```python
from build123d import *

# Parameters (mm, degrees)
SKETCH_1_W                  = 57.4
SKETCH_1_H                  = 28.5
EXTRUDE_1_DEPTH             = 12
SKETCH_2_W                  = 57.4
SKETCH_2_H                  = 26
EXTRUDE_2_DEPTH             = 19
SKETCH_3_W                  = 16.1
SKETCH_3_H                  = 20.5
CUT_EXTRUDE_1_DEPTH         = 7.7
SKETCH_4_W                  = 28.1
SKETCH_4_H                  = 20.5
CUT_EXTRUDE_2_DEPTH         = 41.7
SKETCH_5_W                  = 31
SKETCH_5_H                  = 20.5
CUT_EXTRUDE_3_DEPTH         = 0.3
CUT_EXTRUDE_4_DEPTH         = 2.9
SKETCH_7_W                  = 12
SKETCH_7_H                  = 2.5
CUT_EXTRUDE_5_DEPTH         = 46.4
CUT_EXTRUDE_6_DEPTH         = 7.7
CUT_EXTRUDE_7_DEPTH         = 14.1
CUT_EXTRUDE_8_DEPTH         = 3.3
SKETCH_11_W                 = 11
SKETCH_11_H                 = 12
EXTRUDE_3_DEPTH             = 2.5
SKETCH_12_W                 = 12
SKETCH_12_H                 = 2.75
EXTRUDE_4_DEPTH             = 6
SKETCH_13_W                 = 6
SKETCH_13_H                 = 12
EXTRUDE_5_DEPTH             = 2.5
SKETCH_14_W                 = 12
SKETCH_14_H                 = 5.25
EXTRUDE_6_DEPTH             = 6
SKETCH_15_W                 = 5
SKETCH_15_H                 = 2.5
CUT_EXTRUDE_9_DEPTH         = 45.999333328
SKETCH_16_W                 = 5
SKETCH_16_H                 = 2.5
CUT_EXTRUDE_10_DEPTH        = 45.999333328
SKETCH_17_W                 = 5
SKETCH_17_H                 = 26
EXTRUDE_7_DEPTH             = 2
SKETCH_18_W                 = 10
SKETCH_18_H                 = 6
EXTRUDE_8_DEPTH             = 7
SKETCH_19_W                 = 4
SKETCH_19_H                 = 6.5
HOLE_WIZARD_3_5_3_5_1_D     = 3.5
HOLE_WIZARD_3_5_3_5_1_DEPTH = 12
HOLE_WIZARD_3_5_3_5_2_D     = 3.5
HOLE_WIZARD_3_0_3_3_D       = 3
HOLE_WIZARD_3_0_3_3_DEPTH   = 37.5
HOLE_WIZARD_3_5_3_5_3_D     = 3.5
FILLET_1_R                  = 7
EXTRUDE_START               = -19
SKETCH_28_W                 = 6
SKETCH_28_H                 = 5.25
SKETCH_28_R                 = 1.75
EXTRUDE_9_DEPTH             = 7


with BuildPart() as part:
    # Эскиз1 → Бобышка-Вытянуть1 (new body)
    with BuildSketch(Plane.XY.offset(12)):
        with Locations((0, 1.25)):
            Rectangle(SKETCH_1_W, SKETCH_1_H)
    extrude(amount=-EXTRUDE_1_DEPTH)

    # Эскиз2 → Бобышка-Вытянуть2 (add)
    with BuildSketch(Plane.XY.offset(12)):
        Rectangle(SKETCH_2_W, SKETCH_2_H)
    extrude(amount=EXTRUDE_2_DEPTH)

    # Эскиз3 → Вырез-Вытянуть1 (cut)
    with BuildSketch(Plane.ZY.offset(28.7)):
        with Locations((20.05, 0)):
            Rectangle(SKETCH_3_W, SKETCH_3_H)
    extrude(amount=-CUT_EXTRUDE_1_DEPTH, mode=Mode.SUBTRACT)

    # Эскиз4 → Вырез-Вытянуть2 (cut)
    with BuildSketch(Plane.ZY.offset(21)):
        with Locations((14.05, 0)):
            Rectangle(SKETCH_4_W, SKETCH_4_H)
    extrude(amount=-CUT_EXTRUDE_2_DEPTH, mode=Mode.SUBTRACT)

    # Эскиз5 → Вырез-Вытянуть3 (cut)
    with BuildSketch(Plane.ZY.offset(-20.7)):
        with Locations((15.5, 0)):
            Rectangle(SKETCH_5_W, SKETCH_5_H)
    extrude(amount=-CUT_EXTRUDE_3_DEPTH, mode=Mode.SUBTRACT)

    # Эскиз6 → Вырез-Вытянуть4 (cut)
    with BuildSketch(Plane.XY.offset(31)):
        Polygon((28.7, -13), (28.7, 13), (20.7, 13), (20.7, 10.25), (21, 10.25), (21, -10.25), (20.7, -10.25), (20.7, -13), align=None)
    extrude(amount=-CUT_EXTRUDE_4_DEPTH, mode=Mode.SUBTRACT)

    # Эскиз7 → Вырез-Вытянуть5 (cut)
    with BuildSketch(Plane(origin=(28.7, 0, 0), x_dir=(0, 0, -1), z_dir=(1, 0, 0))):
        with Locations((-6, 14.25)):
            Rectangle(SKETCH_7_W, SKETCH_7_H)
    extrude(amount=-CUT_EXTRUDE_5_DEPTH, mode=Mode.SUBTRACT)

    # Эскиз8 → Вырез-Вытянуть6 (cut)
    with BuildSketch(Plane.ZY.offset(28.7)):
        Polygon((12, -13), (31, -13), (31, 13), (12, 13), (12, 10.25), (28.1, 10.25), (28.1, -10.25), (12, -10.25), align=None)
    extrude(amount=-CUT_EXTRUDE_6_DEPTH, mode=Mode.SUBTRACT)

    # Эскиз9 → Вырез-Вытянуть7 (cut)
    with BuildSketch(Plane.XY.offset(28.1)):
        Polygon((28.7, -13), (28.7, 13), (20.7, 13), (20.7, 10.25), (21, 10.25), (21, -10.25), (20.7, -10.25), (20.7, -13), align=None)
    extrude(amount=-CUT_EXTRUDE_7_DEPTH, mode=Mode.SUBTRACT)

    # Эскиз10 → Вырез-Вытянуть8 (cut)
    with BuildSketch(Plane.ZY.offset(21)):
        Polygon((12, -13), (31, -13), (31, 13), (12, 13), (12, 10.25), (28.1, 10.25), (28.1, -10.25), (12, -10.25), align=None)
    extrude(amount=-CUT_EXTRUDE_8_DEPTH, mode=Mode.SUBTRACT)

    # Эскиз11 → Бобышка-Вытянуть3 (add)
    with BuildSketch(Plane.XZ.offset(13)):
        with Locations((-23.2, 6)):
            Rectangle(SKETCH_11_W, SKETCH_11_H)
    extrude(amount=EXTRUDE_3_DEPTH)

    # Эскиз12 → Бобышка-Вытянуть4 (add)
    with BuildSketch(Plane.ZY.offset(17.7)):
        with Locations((25, -11.625)):
            Rectangle(SKETCH_12_W, SKETCH_12_H)
    extrude(amount=EXTRUDE_4_DEPTH)

    # Эскиз13 → Бобышка-Вытянуть5 (add)
    with BuildSketch(Plane.XZ.offset(13)):
        with Locations((-20.7, 25)):
            Rectangle(SKETCH_13_W, SKETCH_13_H)
    extrude(amount=EXTRUDE_5_DEPTH)

    # Эскиз14 → Бобышка-Вытянуть6 (add)
    with BuildSketch(Plane.ZY.offset(17.7)):
        with Locations((25, 12.875)):
            Rectangle(SKETCH_14_W, SKETCH_14_H)
    extrude(amount=EXTRUDE_6_DEPTH)

    # Эскиз15 → Вырез-Вытянуть9 (cut, through all)
    with BuildSketch(Plane(origin=(0, 0, 0), x_dir=(-1, 0, 0), z_dir=(0, 0, -1))):
        with Locations((26.2, -14.25)):
            Rectangle(SKETCH_15_W, SKETCH_15_H)
    extrude(amount=-CUT_EXTRUDE_9_DEPTH, mode=Mode.SUBTRACT)

    # Эскиз16 → Вырез-Вытянуть10 (cut, through all)
    with BuildSketch(Plane(origin=(0, 0, 0), x_dir=(-1, 0, 0), z_dir=(0, 0, -1))):
        with Locations((26.2, 14.25)):
            Rectangle(SKETCH_16_W, SKETCH_16_H)
    extrude(amount=-CUT_EXTRUDE_10_DEPTH, mode=Mode.SUBTRACT)

    # Эскиз17 → Бобышка-Вытянуть7 (add)
    with BuildSketch(Plane.XY.offset(12)):
        with Locations((-26.2, 0)):
            Rectangle(SKETCH_17_W, SKETCH_17_H)
    extrude(amount=EXTRUDE_7_DEPTH)

    # Эскиз18 → Бобышка-Вытянуть8 (add)
    with BuildSketch(Plane.ZY.offset(28.7)):
        with Locations((5, 0)):
            Rectangle(SKETCH_18_W, SKETCH_18_H)
    extrude(amount=EXTRUDE_8_DEPTH)

    # Эскиз19 → Повернуть1 (revolve)
    with BuildSketch(Plane.XZ, mode=Mode.PRIVATE) as revolve_1_sk:
        with Locations((12.2, 34.25)):
            Rectangle(SKETCH_19_W, SKETCH_19_H)
    revolve(revolve_1_sk.sketch.rotate(Axis((10.2, 0, 37.5), (0, 0, -1)), 180), axis=Axis((10.2, 0, 37.5), (0, 0, -1)))

    # Диаметр отверстия Ø3.5 (3.5)1
    with Locations(Plane.XY.offset(31)):
        with Locations((-20.7, 13), (-20.7, -13)):
            Hole(HOLE_WIZARD_3_5_3_5_1_D / 2, depth=HOLE_WIZARD_3_5_3_5_1_DEPTH)

    # Диаметр отверстия Ø3.5 (3.5)2 (through all)
    with Locations(Plane(origin=(0, 0, 0), x_dir=(-1, 0, 0), z_dir=(0, 0, -1))):
        with Locations((32.7, 0)):
            Hole(HOLE_WIZARD_3_5_3_5_2_D / 2)

    # Диаметр отверстия Ø3.0 (3)3
    with Locations(Plane(origin=(0, 0, 0), x_dir=(-1, 0, 0), z_dir=(0, 0, -1))):
        with Locations((-25.5, -5), (-25.5, 5), (25.5, -5), (25.5, 5)):
            Hole(HOLE_WIZARD_3_0_3_3_D / 2, depth=HOLE_WIZARD_3_0_3_3_DEPTH)

    # Диаметр отверстия Ø3.5 (3.5)3 (through all)
    with Locations(Plane.XY.offset(12)):
        with Locations((-20.7, 13), (-20.7, -13)):
            Hole(HOLE_WIZARD_3_5_3_5_3_D / 2)

    # Скругление1
    fillet_1_edges = [part.edges().sort_by_distance(p)[0] for p in [
        (28.7, 13, 7),
        (28.7, -13, 7),
    ]]
    fillet(fillet_1_edges, radius=FILLET_1_R)

    # Эскиз28 → Бобышка-Вытянуть9 (add)
    # profile 1 of 2: a face of its own
    with BuildSketch(Plane.XY.offset(31).offset(EXTRUDE_START)):
        with Locations((-20.7, 12.875)):
            Rectangle(SKETCH_28_W, SKETCH_28_H)
        with Locations((-20.7, 13)):
            Circle(SKETCH_28_R, mode=Mode.SUBTRACT)
    # profile 2 of 2: a face of its own
    with BuildSketch(Plane.XY.offset(31).offset(EXTRUDE_START)):
        with Locations((-20.7, -12.875)):
            Rectangle(SKETCH_28_W, SKETCH_28_H)
        with Locations((-20.7, -13)):
            Circle(SKETCH_28_R, mode=Mode.SUBTRACT)
    extrude(amount=EXTRUDE_9_DEPTH)


solid = part.part
```
Read the model definition and answer for the solid it produces. Units are mm, in the model's axes. A direction names the side the tool comes from. Coordinates: 2 decimals unless noted, no trailing zeros. Write each loop counter-clockwise with the first axis right and the second up, starting at its lowest first coordinate (ties: lowest second). Pieces come first, ordered by that corner, then holes. Notation, with made-up numbers: (-18, 18.25) - (32, 18.25) arc R17 ccw to (32, 40.25) - close; hole circle Ø1 at (57.25, 45.5). An arc over 180 degrees is marked (long way). Answer as a JSON object with one key per item and string values. Group by question number.
1. Consider L1, parallel to Y at x = -25, z = 4; L2, parallel to Y at x = -14.5, z = 11; L3, parallel to Y at x = 25, z = 11. Determine where each line is inside the solid, lowest interval first. Write a range as [from, to].
2. The mould has two halves that part along Y. Classify faces 1 (the cylindrical face through (-27, 5, 7)), 2 (the flat face through (28.7, 0, 7)), 3 (the flat face through (2, 13, 15)): +Y half, -Y half, draft (parallel to the pull), parting line (faces both ways), or undercut.
3. A cutting plane is placed at A-A (y = 5). Determine the outline of the cut face in (x, z).
4. A cutting plane is placed at B-B (z = 25). Determine the outline of the cut face in (x, y), plus the area to 3 significant figures.
5. A cutting plane is placed at D-D (x = -32.7). Determine the outline of the cut face in (y, z).
6. Which of the six approach directions +Z, -Z, +X, -X, +Y, -Y give full straight-line access (tool end or side, diameter ignored) to faces 4 (the flat face through (-17.7, 0, 30)), 5 (the flat face through (-22, 0, 12)), 6 (the flat face through (1, 0, 28.1))?
7. A cutting plane is placed at C-C (x = -25.5). Determine the outline of the cut face in (y, z), plus the area to 3 significant figures.
8. Each of these flat-tipped pins is pushed along its axis until it touches: P1, Ø0.8, axis at x = -22, y = 2, coming from the +Z side; P2, Ø9, axis at x = 23.5, y = -5.5, coming from the +Z side; P3, Ø1.5, axis at y = -12, z = 10, coming from the -X side; P4, Ø3, axis at x = -20.7, y = -13, coming from the -Z side. Where does it stop, or does it pass through?
Worked out:
{
 "1": {"L1": "y = [-13, -6.41], [-3.59, 3.59], [6.41, 13]", "L2": "y = [-13, -10.25], [10.25, 13]", "L3": "y = [-12.17, -6.41], [-3.59, 3.59], [6.41, 12.17]"},
 "2": {"face 1": "undercut", "face 2": "draft", "face 3": "+Y half"},
 "3": {"outline": "(-28.7, 0) - (-27, 0) - (-27, 14) - (-28.7, 14) - close; (-24, 0) - (-21, 0) - (-21, 12) - (-23.7, 12) - (-23.7, 14) - (-24, 14) - close; (-17.7, 28.1) - (20.7, 28.1) - (20.7, 31) - (-17.7, 31) - close; (21, 0) - (24, 0) - (24, 14) - (21, 14) - close; (27, 0) - (28.7, 0) - (28.7, 14) - (27, 14) - close"},
 "4": {"outline": "(-23.7, -15.5) - (-17.7, -15.5) - (-17.7, -13) - (20.7, -13) - (20.7, -10.25) - (-23.7, -10.25) - close; (-23.7, 10.25) - (20.7, 10.25) - (20.7, 13) - (-17.7, 13) - (-17.7, 15.5) - (-23.7, 15.5) - close; hole circle Ø3.5 at (-20.7, -13); hole circle Ø3.5 at (-20.7, 13)", "area": "255 mm²"},
 "5": {"outline": "(-3, 0) - (-1.75, 0) - (-1.75, 10) - (-3, 10) - close; (1.75, 0) - (3, 0) - (3, 10) - (1.75, 10) - close"},
 "6": {"face 4": "+Z, -Z, -X", "face 5": "+Z", "face 6": "-Z, +X, -X"},
 "7": {"outline": "(-13, 0) - (-6.5, 0) - (-6.5, 14) - (-13, 14) - close; (-3.5, 0) - (3.5, 0) - (3.5, 14) - (-3.5, 14) - close; (6.5, 0) - (13, 0) - (13, 14) - (6.5, 14) - close", "area": "280 mm²"},
 "8": {"P1": "stops at z = 12", "P2": "stops at z = 31", "P3": "stops at x = -28.7", "P4": "passes through"}
}
